from build123d import *

# Parameters (mm, degrees)
CROQUIS1_W              = 50
CROQUIS1_H              = 40
CROQUIS1_R              = 1.75
SALIENTE_EXTRUIR1_DEPTH = 2.5
CROQUIS2_R              = 12.5
CROQUIS2_R_2            = 10
CROQUIS2_R_3            = 8
CROQUIS2_R_4            = 5
SALIENTE_EXTRUIR2_DEPTH = 7
CROQUIS4_R              = 12.5
CROQUIS4_R_2            = 5
SALIENTE_EXTRUIR3_DEPTH = 5
CHAFL_N1_SIZE           = 2


with BuildPart() as part:
    # Croquis1 → Saliente-Extruir1 (new, symmetric)
    with BuildSketch(Plane.XY):
        Rectangle(CROQUIS1_W, CROQUIS1_H)
        with Locations((-20, 16)):
            Circle(CROQUIS1_R, mode=Mode.SUBTRACT)
        with Locations((20, 16)):
            Circle(CROQUIS1_R, mode=Mode.SUBTRACT)
        with Locations((20, -16)):
            Circle(CROQUIS1_R, mode=Mode.SUBTRACT)
        with Locations((-20, -16)):
            Circle(CROQUIS1_R, mode=Mode.SUBTRACT)
    extrude(amount=SALIENTE_EXTRUIR1_DEPTH, both=True)

    # Croquis2 → Saliente-Extruir2 (add)
    with BuildSketch(Plane.XY.offset(2.5)):
        with Locations(Location((0, 0, 0), (0, 0, 180))):
            Circle(CROQUIS2_R)
        Circle(CROQUIS2_R_2, mode=Mode.SUBTRACT)
        with BuildLine():
            ThreePointArc((-9.797958971, 2), (-10, 0), (-9.797958971, -2))
            Line((-9.797958971, -2), (-7.745966692, -2))
            ThreePointArc((-7.745966692, -2), (-8, 0), (-7.745966692, 2))
            Line((-7.745966692, 2), (-9.797958971, 2))
        make_face()
        with BuildLine():
            Line((-5.605034154, -5.708203932), (-6.631030293, -7.485281374))
            ThreePointArc((-6.631030293, -7.485281374), (-5, -8.660254038), (-3.166928678, -9.485281374))
            Line((-3.166928678, -9.485281374), (-2.140932539, -7.708203932))
            ThreePointArc((-2.140932539, -7.708203932), (-4, -6.92820323), (-5.605034154, -5.708203932))
        make_face()
        with BuildLine():
            Line((2.140932539, -7.708203932), (3.166928678, -9.485281374))
            ThreePointArc((3.166928678, -9.485281374), (5, -8.660254038), (6.631030293, -7.485281374))
            Line((6.631030293, -7.485281374), (5.605034154, -5.708203933))
            ThreePointArc((5.605034154, -5.708203933), (4, -6.92820323), (2.140932539, -7.708203932))
        make_face()
        with BuildLine():
            Line((7.745966692, -2), (9.797958971, -2))
            ThreePointArc((9.797958971, -2), (9.94936153, -1.00508962), (10, 0))
            ThreePointArc((10, 0), (9.94936153, 1.00508962), (9.797958971, 2))
            Line((9.797958971, 2), (7.745966692, 2))
            ThreePointArc((7.745966692, 2), (7.93623757, 1.00803434), (8, 0))
            ThreePointArc((8, 0), (7.93623757, -1.00803434), (7.745966692, -2))
        make_face()
        with BuildLine():
            ThreePointArc((6.631030293, 7.485281374), (5, 8.660254038), (3.166928678, 9.485281374))
            Line((3.166928678, 9.485281374), (2.140932539, 7.708203932))
            ThreePointArc((2.140932539, 7.708203932), (4, 6.92820323), (5.605034154, 5.708203932))
            Line((5.605034154, 5.708203932), (6.631030293, 7.485281374))
        make_face()
        with BuildLine():
            ThreePointArc((-3.166928678, 9.485281374), (-5, 8.660254038), (-6.631030293, 7.485281374))
            Line((-6.631030293, 7.485281374), (-5.605034154, 5.708203932))
            ThreePointArc((-5.605034154, 5.708203932), (-4, 6.92820323), (-2.140932539, 7.708203932))
            Line((-2.140932539, 7.708203932), (-3.166928678, 9.485281374))
        make_face()
        Circle(CROQUIS2_R_3)
        Circle(CROQUIS2_R_4, mode=Mode.SUBTRACT)
    extrude(amount=SALIENTE_EXTRUIR2_DEPTH)

    # Croquis4 → Saliente-Extruir3 (add)
    with BuildSketch(Plane.XY.offset(9.5)):
        with Locations(Location((0, 0, 0), (0, 0, 180))):
            Circle(CROQUIS4_R)
        with BuildLine():
            ThreePointArc((9.797958971, 2), (9.94936153, 1.00508962), (10, 0))
            ThreePointArc((10, 0), (9.94936153, -1.00508962), (9.797958971, -2))
            ThreePointArc((9.797958971, -2), (8.660254038, -5), (6.631030293, -7.485281374))
            ThreePointArc((6.631030293, -7.485281374), (5, -8.660254038), (3.166928678, -9.485281374))
            ThreePointArc((3.166928678, -9.485281374), (0, -10), (-3.166928678, -9.485281374))
            ThreePointArc((-3.166928678, -9.485281374), (-5, -8.660254038), (-6.631030293, -7.485281374))
            ThreePointArc((-6.631030293, -7.485281374), (-8.660254038, -5), (-9.797958971, -2))
            ThreePointArc((-9.797958971, -2), (-10, 0), (-9.797958971, 2))
            ThreePointArc((-9.797958971, 2), (-8.660254038, 5), (-6.631030293, 7.485281374))
            ThreePointArc((-6.631030293, 7.485281374), (-5, 8.660254038), (-3.166928678, 9.485281374))
            ThreePointArc((-3.166928678, 9.485281374), (0, 10), (3.166928678, 9.485281374))
            ThreePointArc((3.166928678, 9.485281374), (5, 8.660254038), (6.631030293, 7.485281374))
            ThreePointArc((6.631030293, 7.485281374), (8.660254038, 5), (9.797958971, 2))
        make_face(mode=Mode.SUBTRACT)
        with BuildLine():
            ThreePointArc((7.745966692, -2), (7.93623757, -1.00803434), (8, 0))
            ThreePointArc((8, 0), (7.93623757, 1.00803434), (7.745966692, 2))
            ThreePointArc((7.745966692, 2), (6.92820323, 4), (5.605034154, 5.708203932))
            ThreePointArc((5.605034154, 5.708203932), (4, 6.92820323), (2.140932539, 7.708203932))
            ThreePointArc((2.140932539, 7.708203932), (0, 8), (-2.140932539, 7.708203932))
            ThreePointArc((-2.140932539, 7.708203932), (-4, 6.92820323), (-5.605034154, 5.708203932))
            ThreePointArc((-5.605034154, 5.708203932), (-6.92820323, 4), (-7.745966692, 2))
            ThreePointArc((-7.745966692, 2), (-8, 0), (-7.745966692, -2))
            ThreePointArc((-7.745966692, -2), (-6.92820323, -4), (-5.605034154, -5.708203932))
            ThreePointArc((-5.605034154, -5.708203932), (-4, -6.92820323), (-2.140932539, -7.708203932))
            ThreePointArc((-2.140932539, -7.708203932), (0, -8), (2.140932539, -7.708203932))
            ThreePointArc((2.140932539, -7.708203932), (4, -6.92820323), (5.605034154, -5.708203933))
            ThreePointArc((5.605034154, -5.708203933), (6.92820323, -4), (7.745966692, -2))
        make_face()
        Circle(CROQUIS4_R_2, mode=Mode.SUBTRACT)
    extrude(amount=SALIENTE_EXTRUIR3_DEPTH)

    # Chaflán1
    chafl_n1_edges = [part.edges().sort_by_distance(p)[0] for p in [
        (12.5, 0, 2.5),
    ]]
    chamfer(chafl_n1_edges, length=CHAFL_N1_SIZE)


solid = part.part
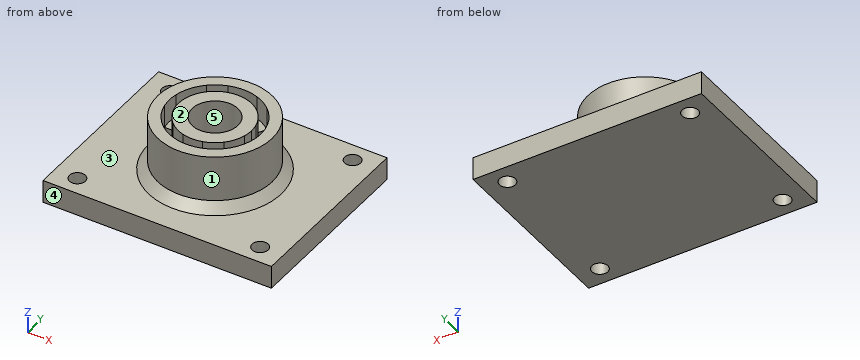
Can you work these out from the model? Positions are in its coordinate system, mm. Face numbers are marked on the shaded views. A direction names the side the tool comes from. Coordinates: 2 decimals unless noted, no trailing zeros. Write each loop counter-clockwise with the first axis right and the second up, starting at its lowest first coordinate (ties: lowest second). Pieces come first, ordered by that corner, then holes.
Q1. Imagine slicing it at C-C, the plane x = -20. List the corners of the cut face in (y, z) for me, plus the area to 3 significant figures.
Results found:
outline: (-20, -2.5) - (-17.75, -2.5) - (-17.75, 2.5) - (-20, 2.5) - close; (-14.25, -2.5) - (14.25, -2.5) - (14.25, 2.5) - (-14.25, 2.5) - close; (17.75, -2.5) - (20, -2.5) - (20, 2.5) - (17.75, 2.5) - close
area: 165 mm2
Q2. Imagine slicing it at D-D, the plane x = 0. List the corners of the cut face in (y, z) for me.
Results found:
outline: (-20, -2.5) - (20, -2.5) - (20, 2.5) - (14.5, 2.5) - (12.5, 4.5) - (12.5, 14.5) - (10, 14.5) - (10, 2.5) - (8, 2.5) - (8, 14.5) - (5, 14.5) - (5, 2.5) - (-5, 2.5) - (-5, 14.5) - (-8, 14.5) - (-8, 2.5) - (-10, 2.5) - (-10, 14.5) - (-12.5, 14.5) - (-12.5, 4.5) - (-14.5, 2.5) - (-20, 2.5) - close
Q3. Which directions (+Z, -Z, +X, -X, +Y, -Y) give clear straight access to the entire face, cutting with the end or side of a thin tool? Please do the marked faces 1 and 2.
Results found:
face 1: +Z
face 2: +Z, +X, -X, +Y, -Y
Q4. Please list where these lines run through material, in increasing order: L1, parallel to Y at x = 20, z = 0.2; L2, parallel to Y at x = 6, z = 13; L3, parallel to X at y = -15, z = 0.25.
Results found:
L1: y = -20 to -17.75, -14.25 to 14.25, 17.75 to 20
L2: y = -10.97 to -8, -5.29 to 5.29, 8 to 10.97
L3: x = -25 to -21.44, -18.56 to 18.56, 21.44 to 25
Q5. Imagine slicing it at B-B, the plane z = -0.75. List the corners of the cut face in (x, y) for me.
Results found:
outline: (-25, -20) - (25, -20) - (25, 20) - (-25, 20) - close; hole circle Ø3.5 at (-20, -16); hole circle Ø3.5 at (-20, 16); hole circle Ø3.5 at (20, -16); hole circle Ø3.5 at (20, 16)
Q6. If we mould it in two halves opening along Y, with no side actions, what happens to the marked faces 3, 4 and 5? For each: +Y half, -Y half, draft (parallel to the pull), parting line (faces both ways), or undercut.
Results found:
face 3: draft
face 4: -Y half
face 5: undercut
Q7. Imagine slicing it at A-A, the plane y = -16. List the corners of the cut face in (x, z) for me.
Results found:
outline: (-25, -2.5) - (-21.75, -2.5) - (-21.75, 2.5) - (-25, 2.5) - close; (-18.25, -2.5) - (18.25, -2.5) - (18.25, 2.5) - (-18.25, 2.5) - close; (21.75, -2.5) - (25, -2.5) - (25, 2.5) - (21.75, 2.5) - close
Q8. For P1, Ø4.5, axis at x = 7.5, y = -5, coming from the +Z side; P2, Ø3, axis at x = 5.5, z = 5, coming from the +Y side; P3, Ø3, axis at y = 7, z = 10.5, coming from the -X side (3 decimals); P4, Ø1, axis at x = -8.5, z = 11.5, coming from the -Y side, each with a flat end and sliding along its axis, tell me the tip position at first contact or that it passes through.
Results found:
P1: stops at z = 14.5
P2: stops at y = 12.45
P3: stops at x = -11.225
P4: stops at y = -9.6
